Read the model definition and answer for the solid it produces. Units are mm, in the model's axes. A direction names the side the tool comes from. Coordinates: 2 decimals unless noted, no trailing zeros. Loops run counter-clockwise (first coordinate to the right, second up) from the corner with the lowest first, then second, coordinate; pieces in that order, holes last.
from build123d import *

# Parameters (mm, degrees)
SKETCH1_W           = 6
SKETCH1_H           = 197
SKETCH1_R           = 1.55
SKETCH1_H_2         = 3
BOSS_EXTRUDE1_DEPTH = 106
SKETCH2_W           = 6
SKETCH2_H           = 33
CUT_EXTRUDE1_DEPTH  = 234
FILLET2_R           = 10
SKETCH2_5_W         = 5
SKETCH2_5_H         = 3
SKETCH2_5_W_2       = 103.95
SKETCH2_5_W_3       = 8.1
CUT_EXTRUDE2_DEPTH  = 198
FILLET1_R           = 35


with BuildPart() as part:
    # Sketch1 → Boss-Extrude1 (new body)
    # profile 1 of 7: a face of its own
    with BuildSketch(Plane.XY):
        with Locations((225, 101.5)):
            Rectangle(SKETCH1_W, SKETCH1_H)
        with Locations((225, 27.25)):
            Circle(SKETCH1_R, mode=Mode.SUBTRACT)
        with Locations((225, 51.5)):
            Circle(SKETCH1_R, mode=Mode.SUBTRACT)
        with Locations((225, 75.75)):
            Circle(SKETCH1_R, mode=Mode.SUBTRACT)
        with Locations((225, 100)):
            Circle(SKETCH1_R, mode=Mode.SUBTRACT)
        with Locations((225, 124.25)):
            Circle(SKETCH1_R, mode=Mode.SUBTRACT)
        with Locations((225, 148.5)):
            Circle(SKETCH1_R, mode=Mode.SUBTRACT)
        with Locations((225, 172.75)):
            Circle(SKETCH1_R, mode=Mode.SUBTRACT)
    # profile 2 of 7: a face of its own
    with BuildSketch(Plane.XY):
        Polygon((178.113248654, -1), (178.113248654, 0), (163.886751346, 0), (163.886751346, -1), (161, -6), (181, -6), align=None)
    # profile 3 of 7: a face of its own
    with BuildSketch(Plane.XY):
        Polygon((64.113248654, 0), (49.886751346, 0), (49.886751346, -1), (47, -6), (67, -6), (64.113248654, -1), align=None)
    # profile 4 of 7: a face of its own
    with BuildSketch(Plane.XY):
        Polygon((222, 3), (6, 3), (6, 0), (49.886751346, 0), (64.113248654, 0), (163.886751346, 0), (178.113248654, 0), (222, 0), align=None)
    # profile 5 of 7: a face of its own
    with BuildSketch(Plane.XY):
        with Locations((225, 1.5)):
            Rectangle(SKETCH1_W, SKETCH1_H_2)
    # profile 6 of 7: a face of its own
    with BuildSketch(Plane.XY):
        with Locations((3, 1.5)):
            Rectangle(SKETCH1_W, SKETCH1_H_2)
    # profile 7 of 7: a face of its own
    with BuildSketch(Plane.XY):
        with Locations((3, 101.5)):
            Rectangle(SKETCH1_W, SKETCH1_H)
        with Locations((3, 27.25)):
            Circle(SKETCH1_R, mode=Mode.SUBTRACT)
        with Locations((3, 51.5)):
            Circle(SKETCH1_R, mode=Mode.SUBTRACT)
        with Locations((3, 75.75)):
            Circle(SKETCH1_R, mode=Mode.SUBTRACT)
        with Locations((3, 100)):
            Circle(SKETCH1_R, mode=Mode.SUBTRACT)
        with Locations((3, 124.25)):
            Circle(SKETCH1_R, mode=Mode.SUBTRACT)
        with Locations((3, 148.5)):
            Circle(SKETCH1_R, mode=Mode.SUBTRACT)
        with Locations((3, 172.75)):
            Circle(SKETCH1_R, mode=Mode.SUBTRACT)
    extrude(amount=BOSS_EXTRUDE1_DEPTH)

    # Sketch2 → Cut-Extrude1 (cut)
    with BuildSketch(Plane(origin=(0, 200, 0), x_dir=(1, 0, 0), z_dir=(0, 1, 0))):
        with BuildLine():
            Line((109.95, -20), (109.95, -50))
            Line((109.95, -50), (118.05, -50))
            Line((118.05, -50), (118.05, -20))
            ThreePointArc((118.05, -20), (114, -15.95), (109.95, -20))
        make_face()
        with BuildLine():
            Line((118.05, -56), (109.95, -56))
            Line((109.95, -56), (109.95, -86))
            ThreePointArc((109.95, -86), (114, -90.05), (118.05, -86))
            Line((118.05, -86), (118.05, -56))
        make_face()
        with Locations((225, -89.5)):
            Rectangle(SKETCH2_W, SKETCH2_H)
        with Locations((225, -16.5)):
            Rectangle(SKETCH2_W, SKETCH2_H)
        with Locations((3, -16.5)):
            Rectangle(SKETCH2_W, SKETCH2_H)
        with Locations((3, -89.5)):
            Rectangle(SKETCH2_W, SKETCH2_H)
    extrude(amount=-CUT_EXTRUDE1_DEPTH, mode=Mode.SUBTRACT)

    # Fillet2
    fillet2_edges = [part.edges().sort_by_distance(p)[0] for p in [
        (228, 0, 53),
        (222, 3, 53),
        (0, 0, 53),
        (6, 3, 53),
    ]]
    fillet(fillet2_edges, radius=FILLET2_R)

    # Sketch2<5> → Cut-Extrude2 (cut)
    with BuildSketch(Plane(origin=(0, 200, 0), x_dir=(1, 0, 0), z_dir=(0, 1, 0))):
        with Locations((224.5, -53)):
            Rectangle(SKETCH2_5_W, SKETCH2_5_H)
        with Locations((170.025, -53)):
            Rectangle(SKETCH2_5_W_2, SKETCH2_5_H)
        with Locations((57.975, -53)):
            Rectangle(SKETCH2_5_W_2, SKETCH2_5_H)
        with Locations((114, -53)):
            Rectangle(SKETCH2_5_W_3, SKETCH2_5_H)
        with Locations((3.5, -53)):
            Rectangle(SKETCH2_5_W, SKETCH2_5_H)
    extrude(amount=-CUT_EXTRUDE2_DEPTH, mode=Mode.SUBTRACT)

    # Fillet1
    # the kernel refuses this fillet: 35 mm, written as the material it takes off along each edge
    with BuildSketch(Plane(origin=(222, 90.357026048, 0), x_dir=(0, 0, 1), z_dir=(0, -1, 0))) as fillet1_piece_1:
        with BuildLine():
            CenterArc((35, 34.942810419), FILLET1_R, 180, 86.72417104)
            Line((0, 34.942810419), (-0.7, 34.942810419))
            Line((-0.7, 34.942810419), (-0.7, 0))
            Line((-0.7, 0), (0, -0.7))
            ThreePointArc((0, -0.7), (16.5, -0.7), (32.96, -0.698856208))
            Line((32.96, -0.698856208), (33, 0))
        make_face()
    extrude(amount=176.879203486, mode=Mode.SUBTRACT)
    with BuildSketch(Plane(origin=(6, 90.357026048, 0), x_dir=(1, 0, 0), z_dir=(0, -1, 0)), Plane(origin=(222, 90.357026048, 106), x_dir=(-1, 0, 0), z_dir=(0, -1, 0))) as fillet1_piece_2:
        with BuildLine():
            CenterArc((34.942810419, 35), FILLET1_R, 183.27582896, 86.72417104)
            Line((0, 33), (-0.698856208, 32.96))
            ThreePointArc((-0.698856208, 32.96), (-0.7, 16.5), (-0.7, 0))
            Line((-0.7, 0), (0, -0.7))
            Line((0, -0.7), (34.942810419, -0.7))
            Line((34.942810419, -0.7), (34.942810419, 0))
        make_face()
    extrude(amount=176.879203486, mode=Mode.SUBTRACT)
    with BuildSketch(Plane(origin=(6, 90.357026048, 106), x_dir=(1, 0, 0), z_dir=(0, -1, 0))) as fillet1_piece_3:
        with BuildLine():
            CenterArc((34.942810419, -35), FILLET1_R, 90, 86.72417104)
            Line((0, -33), (-0.698856208, -32.96))
            ThreePointArc((-0.698856208, -32.96), (-0.7, -16.5), (-0.7, 0))
            Line((-0.7, 0), (0, 0.7))
            Line((0, 0.7), (34.942810419, 0.7))
            Line((34.942810419, 0.7), (34.942810419, 0))
        make_face()
    extrude(amount=176.879203486, mode=Mode.SUBTRACT)


solid = part.part
Item 1: Find the intervals of material crossed by line 1 along X through (y, z) = (100, 64.5); line 2 along X through (y, z) = (114, 66); line 3 along Y through (x, z) = (37, 78), in increasing order.
Numbers:
line 1: x = 0 to 1.45, 4.55 to 6, 222 to 223.45, 226.55 to 228
line 2: x = 0 to 6, 222 to 228
line 3: y = 0 to 3
Item 2: Which of the six approach directions +Z, -Z, +X, -X, +Y, -Y give full straight-line access (tool end or side, diameter ignored) to faces 1 (the face through (65.577, -3.535, 52.258)), 2 (the face through (218.99, 5.85, 42.38)), 3 (the face through (223, 101, 51.5))?
Numbers:
face 1: +Z, -Z
face 2: +Z, -Z, +Y
face 3: +Y
Item 3: A cutting plane is placed at D-D on x = 169.5. Determine the outline of the cut face in (y, z), then the cut area to 3 significant figures.
Numbers:
outline: (-6, 0) - (3, 0) - (3, 51.5) - (2, 51.5) - (2, 54.5) - (3, 54.5) - (3, 106) - (-6, 106) - close
area: 951 mm2
Item 4: Determine the mould class of faces 4 (the face through (198, 0, 52)), 5 (the face through (116, 3, 14)), 6 (the face through (0, 104, 53)) for opening direction X: released by +X, released by -X, zero draft, split by the parting line, or undercut.
Numbers:
face 4: zero draft
face 5: undercut
face 6: released by -X
Item 5: A cutting plane is placed at C-C on z = 11.5. Determine the outline of the cut face in (x, y), then the cut area to 3 significant figures.
Numbers:
outline: (15.01, 0) - (49.89, 0) - (49.89, -1) - (47, -6) - (67, -6) - (64.11, -1) - (64.11, 0) - (163.89, 0) - (163.89, -1) - (161, -6) - (181, -6) - (178.11, -1) - (178.11, 0) - (212.99, 0) - (212.99, 3) - (15.01, 3) - close
area: 794 mm2
Item 6: A cutting plane is placed at A-A on y = 34.5. Determine the outline of the cut face in (x, z).
Numbers:
outline: (0, 33) - (6, 33) - (6, 51.5) - (1, 51.5) - (1, 54.5) - (6, 54.5) - (6, 73) - (0, 73) - close; (222, 33) - (228, 33) - (228, 73) - (222, 73) - (222, 54.5) - (227, 54.5) - (227, 51.5) - (222, 51.5) - close
Item 7: Given pin 1 (4 mm diameter, centred on x = 225, y = 124.25, fed in from -Z); pin 2 (5 mm diameter, centred on x = 188, z = 33.5, fed in from +Y); pin 3 (0.9 mm diameter, centred on y = 1, z = 38.5, fed in from -X); pin 4 (3.5 mm diameter, centred on x = 114, y = 1, fed in from -Z), each flat-ended and moving along its own axis, determine where each tip first touches the part or whether it passes through.
Numbers:
pin 1: stops at z = 33
pin 2: stops at y = 3
pin 3: stops at x = 4.81
pin 4: stops at z = 0
Item 8: A cutting plane is placed at B-B on x = 102. Determine the outline of the cut face in (y, z), then the cut area to 3 significant figures.
Numbers:
outline: (0, 0) - (3, 0) - (3, 51.5) - (2, 51.5) - (2, 54.5) - (3, 54.5) - (3, 106) - (0, 106) - close
area: 315 mm2
